Print and shaded views of the part. All mm, measured from the part's lowest x, y and z. Give positions to 0.01 mm unless a question says otherwise; leave off trailing zeros. Order: outer loops, then holes, each group sorted by start corner. A loop starts at its lowest first (then second) coordinate and runs counter-clockwise, first axis right, second up. Notation, with made-up numbers: (82, -1) -> (86, -1) arc R27 cw to (86, 21) -> close; hole circle Ø9 at (77, 4.5). An arc over 180 degrees is marked (long way). One line per question, with ' | ' between items. Start each with the question number.
(1) Pin check, flat tips, straight feed: pin 1 Ø3 at (y, z) = (3.5, 35.5) entering from +X; pin 2 Ø1.5 at (x, y) = (109.5, 0.5) entering from -Z; pin 3 Ø1 at (y, z) = (4.5, 95.5) entering from +X. Stop position of each tip, or through.
(2) Cut at B-B (z = 154.5). Give the cut face in (x, y).
(3) Drill centre lines: L1, parallel to X at y = 4, z = 109.5 (1 decimal); L2, parallel to X at y = 5, z = 187 (1 decimal); L3, parallel to Z at x = 213.5, y = 4.25. Where is each one in solid material? Low to high. Write a range as from..to.
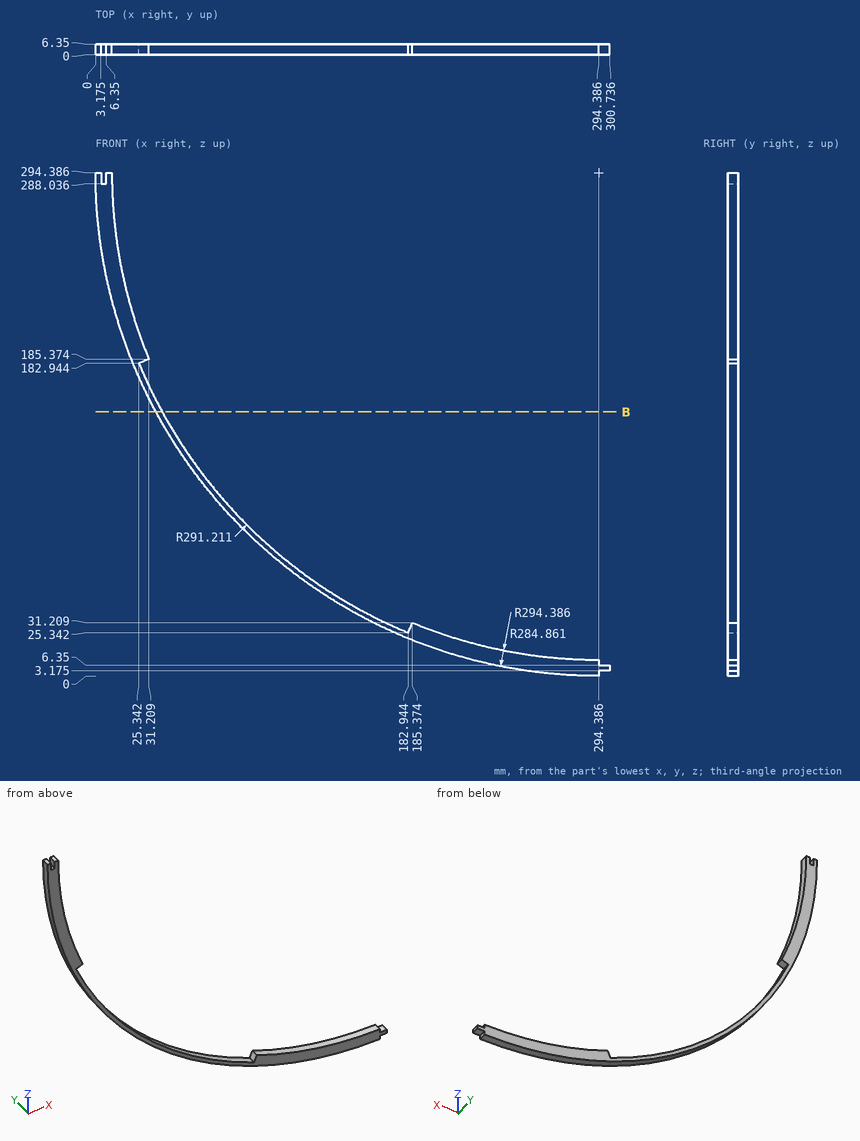
Result set:
1) pin 1: stops at x = 163.99 | pin 2: stops at z = 64.7 | pin 3: stops at x = 82.14
2) outline: (35.36, 0) -> (38.97, 0) -> (38.97, 6.35) -> (35.36, 6.35) -> close
3) L1: x = 65.3..69.4 | L2: x = 20.3..30.5 | L3: z = 11.33..21.25
